from build123d import *

# Parameters (mm, degrees)
SKETCH_1_W          = 10
SKETCH_1_H          = 40
SKETCH_1_R          = 3.5
EXTRUDE_1_DEPTH     = 10
SKETCH_2_R          = 1.5
CUT_EXTRUDE_1_DEPTH = 25.494897428


with BuildPart() as part:
    # 草图1 → 凸台-拉伸1 (new body)
    with BuildSketch(Plane.XY):
        Rectangle(SKETCH_1_W, SKETCH_1_H)
        with Locations((0, 13)):
            Circle(SKETCH_1_R, mode=Mode.SUBTRACT)
        with Locations((0, -13)):
            Circle(SKETCH_1_R, mode=Mode.SUBTRACT)
    extrude(amount=EXTRUDE_1_DEPTH)

    # 草图2 → 切除-拉伸1 (cut, through all)
    with BuildSketch(Plane(origin=(5, 0, 0), x_dir=(0, 0, -1), z_dir=(1, 0, 0))):
        with Locations(Location((-5, 5, 0), (0, 0, 90))):
            Circle(SKETCH_2_R)
        with Locations(Location((-5, -5, 0), (0, 0, 90))):
            Circle(SKETCH_2_R)
        with Locations(Location((-2.5, 0, 0), (0, 0, 90))):
            Circle(SKETCH_2_R)
        with Locations(Location((-7.5, 0, 0), (0, 0, 90))):
            Circle(SKETCH_2_R)
    extrude(amount=-CUT_EXTRUDE_1_DEPTH, mode=Mode.SUBTRACT)


solid = part.part
Read the model definition and answer for the solid it produces. Units are mm, in the model's axes. Give positions to 0.01 mm unless a question says otherwise; leave off trailing zeros. Write each loop counter-clockwise with the first axis right and the second up, starting at its lowest first coordinate (ties: lowest second). Pieces come first, ordered by that corner, then holes. Notation, with made-up numbers: (-34.75, 26) - (-13.75, 26) arc R36 ccw to (-13.75, 63) - close; hole circle Ø5 at (76.5, 12.25). An arc over 180 degrees is marked (long way). Answer in a Markdown table with one row per item. Add a question column.
Item 1: Find the intervals of material crossed by L1, parallel to Z at x = 0.25, y = 0; L2, parallel to Z at x = -0.75, y = -5; L3, parallel to Y at x = 1.5, z = 2.25, in increasing order.
Item 2: A flat-ended cylindrical pin translates along its axis: P1, Ø2.5, axis at y = 0, z = 2.5, coming from the +X side. Find the tip coordinate at first contact, or state that the pin passes through.
Item 3: Section C-C, the plane y = -5 is taken. Write down the section's boundary in (x, z).
Item 4: Determine the mould class of faces 1 (the face through (0, 0, 0)), 2 (the face through (0, 20, 5)), 3 (the face through (0.07, -6.5, 5.07)) for opening direction Z: pulls with the +Z half, pulls with the -Z half, needs draft (parallel to the pull), parting line crosses it, or undercut.
Item 5: Section B-B, the plane x = 0 is taken. Write down the section's boundary in (y, z), and give its area (3 significant figures).
Item 6: Section D-D, the plane x = 4.5 is taken. Write down the section's boundary in (y, z).
Item 7: Section A-A, the plane z = 5 is taken. Write down the section's boundary in (x, y), and give its area (3 significant figures).
Recorded:
| question | item | result |
|---|---|---|
| 1 | L1 | z = 0 to 1, 4 to 6, 9 to 10 |
| 1 | L2 | z = 0 to 3.5, 6.5 to 10 |
| 1 | L3 | y = -20 to -16.16, -9.84 to -1.48, 1.48 to 9.84, 16.16 to 20 |
| 2 | P1 | passes through |
| 3 | outline | (-5, 0) - (5, 0) - (5, 3.5) - (-5, 3.5) - close; (-5, 6.5) - (5, 6.5) - (5, 10) - (-5, 10) - close |
| 4 | face 1 | pulls with the -Z half |
| 4 | face 2 | needs draft |
| 4 | face 3 | undercut |
| 5 | outline | (-20, 0) - (-16.5, 0) - (-16.5, 10) - (-20, 10) - close; (-9.5, 0) - (9.5, 0) - (9.5, 10) - (-9.5, 10) - close; (16.5, 0) - (20, 0) - (20, 10) - (16.5, 10) - close; hole circle Ø3 at (-5, 5); hole circle Ø3 at (0, 2.5); hole circle Ø3 at (0, 7.5); hole circle Ø3 at (5, 5) |
| 5 | area | 232 mm2 |
| 6 | outline | (-20, 0) - (20, 0) - (20, 10) - (-20, 10) - close; hole circle Ø3 at (-5, 5); hole circle Ø3 at (0, 2.5); hole circle Ø3 at (0, 7.5); hole circle Ø3 at (5, 5) |
| 7 | outline | (-5, -20) - (5, -20) - (5, -6.5) - (-5, -6.5) - close; (-5, -3.5) - (5, -3.5) - (5, 3.5) - (-5, 3.5) - close; (-5, 6.5) - (5, 6.5) - (5, 20) - (-5, 20) - close; hole circle Ø7 at (0, -13); hole circle Ø7 at (0, 13) |
| 7 | area | 263 mm2 |
